Work out the finished part from the listing and answer in its coordinate system (mm). A direction names the side the tool comes from. Give positions to 0.01 mm unless a question says otherwise; leave off trailing zeros. Loops run counter-clockwise (first coordinate to the right, second up) from the corner with the lowest first, then second, coordinate; pieces in that order, holes last. Notation, with made-up numbers: M 73.25,39 L 110.25,39 A25 ccw 110.25,74 Z; hole C 16,22.25 d4. An arc over 180 degrees is marked long. Write item = value, one per line. Start each with the question number.
1. Section D-D on y = -23 is taken. Determine the outline of the cut face in (x, z).
2. Section A-A on z = -5.75 is taken. Determine the outline of the cut face in (x, y), plus the area to 3 significant figures.
3. For faces 4 (the face through (28.263, -25.614, 13.882)), 5 (the face through (9, 0, 4)), 6 (the face through (47, -13, -0.725)), 7 (the face through (10, -13, -7.344)), determine the directions among +Z, -Z, +X, -X, +Y, -Y from which every point of the face is accessible in a straight line to the end or side of a thin tool.
4. Consider L1, parallel to X at y = -21.75, z = -6.25; L2, parallel to Y at x = 9, z = 5.5; L3, parallel to Z at x = -15.5, y = -7.75. Determine where each line is inside the solid, lowest interval first. Write a range as [from, to].
5. Section B-B on x = 14.5 is taken. Determine the outline of the cut face in (y, z).
6. Flat-ended cylindrical pins translate along their axes: pin 1 Ø1 at (y, z) = (-3, 10) entering from +X; pin 2 Ø4 at (x, y) = (-11, -19) entering from +Z; pin 3 Ø0.6 at (x, y) = (46.5, -11.5) entering from +Z. Find the tip coordinate at first contact, or state that the pin passes through.
7. Section C-C on z = 2.25 is taken. Determine the outline of the cut face in (x, y).
8. The mould has two halves that part along X. Classify faces 1 (the face through (36, -26, 17.656)), 2 (the face through (-27.511, -13, 4)), 3 (the face through (22.32, -25.61, 12.1)): released by +X, released by -X, zero draft, split by the parting line, or undercut.
```python
from build123d import *

# Parameters (mm, degrees)
F0_R     = 1.6228665853
F0_R_2   = 1.5
F0_W     = 2
F0_H     = 25
F1_DEPTH = 2
F2_DEPTH = 25.6
F3_DEPTH = 24.6


with BuildPart() as f1:
    # F0 (on Front) → F1 (new body)
    with BuildSketch(Plane.XZ):
        with BuildLine():
            Line((47.4890847677, -0.7248306477), (47.4890847677, 6.2918234199))
            Line((47.4890847677, 6.2918234199), (47.4890847677, 17.6555038384))
            Line((47.4890847677, 17.6555038384), (23.7640682912, 17.6555038384))
            Line((23.7640682912, 17.6555038384), (32.8890847677, 10.0022964448))
            ThreePointArc((32.8890847677, 10.0022964448), (35.6455609426, 1.7196562102), (28.4755586515, 6.6987482262))
            Line((28.4755586515, 6.6987482262), (15.9851853108, 17.6555038384))
            Line((15.9851853108, 17.6555038384), (-5.2803540298, 17.6555038384))
            Line((-5.2803540298, 17.6555038384), (-25.5109152323, 17.6555038384))
            Line((-25.5109152323, 17.6555038384), (-25.5109152323, -7.3444961616))
            Line((-25.5109152323, -7.3444961616), (1.1948530817, -7.3444961616))
            Line((1.1948530817, -7.3444961616), (45.4890847677, -7.3444961616))
            Line((45.4890847677, -7.3444961616), (45.4890847677, -0.7248306477))
            Line((45.4890847677, -0.7248306477), (47.4890847677, -0.7248306477))
        make_face()
        with Locations((13.761951353, -2.5673627469)):
            Circle(F0_R, mode=Mode.SUBTRACT)
        with Locations((13.761951353, 15.1555038384)):
            Circle(F0_R_2, mode=Mode.SUBTRACT)
        Polygon((47.4890847677, -9.3444961616), (47.4890847677, -0.7248306477), (45.4890847677, -0.7248306477), (45.4890847677, -7.3444961616), (45.4890847677, -9.3444961616), align=None)
        Polygon((5.9280249222, -9.3444961616), (45.4890847677, -9.3444961616), (45.4890847677, -7.3444961616), (1.1948530817, -7.3444961616), (-25.5109152323, -7.3444961616), (-27.5109152323, -7.3444961616), (-27.5109152323, -9.3444961616), align=None)
        with Locations((-26.5109152323, 5.1555038384)):
            Rectangle(F0_W, F0_H)
    extrude(amount=F1_DEPTH)

    # F0 (on Front) → F2 (join)
    with BuildSketch(Plane.XZ):
        Polygon((47.4890847677, -9.3444961616), (47.4890847677, -0.7248306477), (45.4890847677, -0.7248306477), (45.4890847677, -7.3444961616), (45.4890847677, -9.3444961616), align=None)
        Polygon((5.9280249222, -9.3444961616), (45.4890847677, -9.3444961616), (45.4890847677, -7.3444961616), (1.1948530817, -7.3444961616), (-25.5109152323, -7.3444961616), (-27.5109152323, -7.3444961616), (-27.5109152323, -9.3444961616), align=None)
    extrude(amount=F2_DEPTH)

    # F0 (on Front) → F3 (join)
    with BuildSketch(Plane.XZ):
        with Locations((-26.5109152323, 5.1555038384)):
            Rectangle(F0_W, F0_H)
    extrude(amount=F3_DEPTH)

    # F5: F1 across plane


with BuildPart() as f1_1:
    add(f1.part)
    add(f1.part.mirror(Plane.XZ.offset(13.3)))


solid = f1_1.part
```
Verdict:
q1.outline = M -27.51,-9.34 L 47.49,-9.34 L 47.49,-0.72 L 45.49,-0.72 L 45.49,-7.34 L -25.51,-7.34 L -25.51,17.66 L -27.51,17.66 Z
q2.outline = M -27.51,-26.6 L 47.49,-26.6 L 47.49,0 L -27.51,0 Z; hole M -25.51,-24.6 L 45.49,-24.6 L 45.49,-2 L -25.51,-2 Z
q2.area = 390 mm2
q3.face_4 = +Y, -Y
q3.face_5 = +Z, -Z, +X, -X, +Y
q3.face_6 = +Z, +X
q3.face_7 = +Z
q4.L1 = [-27.51, -25.51], [45.49, 47.49]
q4.L2 = [-26.6, -24.6], [-2, 0]
q4.L3 = [-9.34, -7.34]
q5.outline = M -26.6,-9.34 L 0,-9.34 L 0,-4.01 L -2,-4.01 L -2,-7.34 L -24.6,-7.34 L -24.6,-4.01 L -26.6,-4.01 Z; M -26.6,-1.12 L -24.6,-1.12 L -24.6,13.85 L -26.6,13.85 Z; M -26.6,16.46 L -24.6,16.46 L -24.6,17.66 L -26.6,17.66 Z; M -2,-1.12 L 0,-1.12 L 0,13.85 L -2,13.85 Z; M -2,16.46 L 0,16.46 L 0,17.66 L -2,17.66 Z
q6.pin_1 = -25.51
q6.pin_2 = -7.34
q6.pin_3 = -0.72
q7.outline = M -27.51,-26.6 L 29.54,-26.6 L 29.54,-24.6 L -25.51,-24.6 L -25.51,-2 L 29.54,-2 L 29.54,0 L -27.51,0 Z; M 36.24,-26.6 L 47.49,-26.6 L 47.49,-24.6 L 36.24,-24.6 Z; M 36.24,-2 L 47.49,-2 L 47.49,0 L 36.24,0 Z
q8.face_1 = zero draft
q8.face_2 = released by -X
q8.face_3 = undercut
